The listing builds one solid part. Answer for the finished solid, in the listing's coordinates (mm). Face numbers are marked on the shaded views. A direction names the side the tool comes from. Give positions to 0.01 mm unless a question says otherwise; leave off trailing zeros. Loops run counter-clockwise (first coordinate to the right, second up) from the corner with the lowest first, then second, coordinate; pieces in that order, holes last. Notation, with made-up numbers: (35.25, 0.5) - (78.25, 0.5) arc R27 cw to (78.25, 37.5) - close; hole circle Ø5 at (0, 58.25). An arc over 180 degrees is marked (long way). Answer in a Markdown table with one row per item. Add a question column.
```python
from build123d import *

# Parameters (mm, degrees)
CROQUIS4_R            = 1.7
CORTAR_EXTRUIR1_DEPTH = 10
CORTAR_EXTRUIR2_DEPTH = 2.5


with BuildPart() as part:
    # Croquis1 → Revolución1 (revolve)
    with BuildSketch(Plane.XY):
        with BuildLine():
            Line((50, 12), (36, 12))
            Line((36, 12), (36, 8.039736831))
            ThreePointArc((36, 8.039736831), (38.2, 5), (36, 1.960263169))
            Line((36, 1.960263169), (36, 0))
            Line((36, 0), (40, 0))
            Line((40, 0), (40, 5))
            Line((40, 5), (50, 5))
            Line((50, 5), (50, 12))
        make_face()
    revolve(axis=Axis((0, 9.671658493, 0), (0, -1, 0)))

    # Croquis2 → Cortar-Revolución1 (revolve, cut)
    with BuildSketch(Plane(origin=(0, 5, 0), x_dir=(1, 0, 0), z_dir=(0, 1, 0))):
        Polygon((-35.5, 0), (-51.5, 0), (-51.5, 3.7), (-40.5, 3.7), (-35.5, 3), align=None)
    revolve(axis=Axis((-54.955446394, 5, 0), (1, 0, 0)), mode=Mode.SUBTRACT)

    # Croquis4 → Cortar-Extruir1 (cut)
    with BuildSketch(Plane(origin=(0, 12, 0), x_dir=(1, 0, 0), z_dir=(0, 1, 0))):
        with Locations((-39, 22.5)):
            Circle(CROQUIS4_R)
        with Locations((39, 22.5)):
            Circle(CROQUIS4_R)
        with Locations((39, -22.5)):
            Circle(CROQUIS4_R)
        with Locations((-39, -22.5)):
            Circle(CROQUIS4_R)
    extrude(amount=-CORTAR_EXTRUIR1_DEPTH, mode=Mode.SUBTRACT)

    # Croquis5 → Cortar-Extruir2 (cut)
    with BuildSketch(Plane(origin=(0, 12, 0), x_dir=(1, 0, 0), z_dir=(0, 1, 0))):
        Polygon((-42.35, 22.5), (-40.675, 19.598814897), (-37.325, 19.598814897), (-35.65, 22.5), (-37.325, 25.401185103), (-40.675, 25.401185103), align=None)
        Polygon((-42.35, -22.5), (-40.675, -25.401185103), (-37.325, -25.401185103), (-35.65, -22.5), (-37.325, -19.598814897), (-40.675, -19.598814897), align=None)
        Polygon((35.65, 22.5), (37.325, 19.598814897), (40.675, 19.598814897), (42.35, 22.5), (40.675, 25.401185103), (37.325, 25.401185103), align=None)
        Polygon((35.65, -22.5), (37.325, -25.401185103), (40.675, -25.401185103), (42.35, -22.5), (40.675, -19.598814897), (37.325, -19.598814897), align=None)
    extrude(amount=-CORTAR_EXTRUIR2_DEPTH, mode=Mode.SUBTRACT)


solid = part.part
```
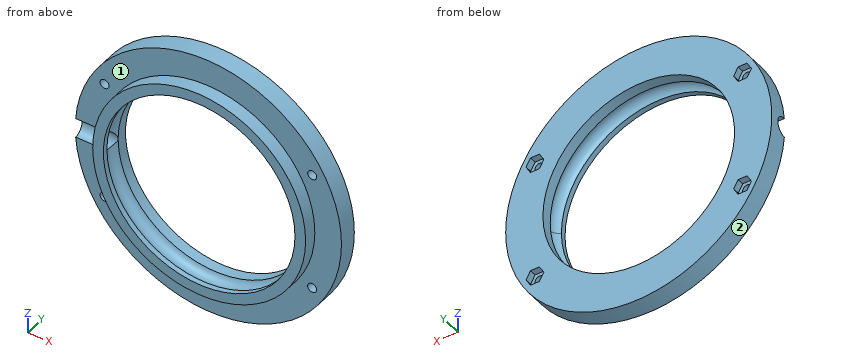
(1) A cutting plane is placed at A-A on x = 0. Determine the outline of the cut face in (y, z), plus the area to 3 significant figures.
(2) A tool of negligible diameter and unlimited length cuts with its end or side. For the marked faces 1 and 2, from which of +Z, -Z, +X, -X, +Y, -Y can it reach the whole face along a straight path? Write none if from no direction.
(3) Given pin 1 Ø0.8 at (x, y) = (-39.5, 10.5) entering from -Z; pin 2 Ø4.5 at (x, z) = (-39, 22.5) entering from +Y; pin 3 Ø2 at (y, z) = (3.5, 30) entering from +X; pin 4 Ø6.5 at (x, z) = (39, 21.5) entering from +Y, each flat-ended and moving along its own axis, determine where each tip first touches the part or whether it passes through.
(4) Find the intervals of material crossed by line 1 along X through (y, z) = (8.4, -22.5); line 2 along X through (y, z) = (6.8, 22.5); line 3 along Y through (x, z) = (-11.5, -41), in increasing order. Write a range as [from, to].
Evaluation:
| question | item | result |
|---|---|---|
| 1 | outline | (0, -40) - (5, -40) - (5, -50) - (12, -50) - (12, -36) - (8.04, -36) arc R3.2 cw to (1.96, -36) - (0, -36) - close; (0, 36) - (1.96, 36) arc R3.2 cw to (8.04, 36) - (12, 36) - (12, 50) - (5, 50) - (5, 40) - (0, 40) - close |
| 1 | area | 216 mm² |
| 2 | face 1 | -Y |
| 2 | face 2 | +Y, -Y |
| 3 | pin 1 | stops at z = -31.16 |
| 3 | pin 2 | stops at y = 9.5 |
| 3 | pin 3 | stops at x = 27.55 |
| 3 | pin 4 | stops at y = 12 |
| 4 | line 1 | x = [-44.65, -40.7], [-37.3, -28.1], [28.1, 37.3], [40.7, 44.65] |
| 4 | line 2 | x = [-44.65, -40.7], [-37.3, -30.18], [30.18, 37.3], [40.7, 44.65] |
| 4 | line 3 | y = [5, 12] |
